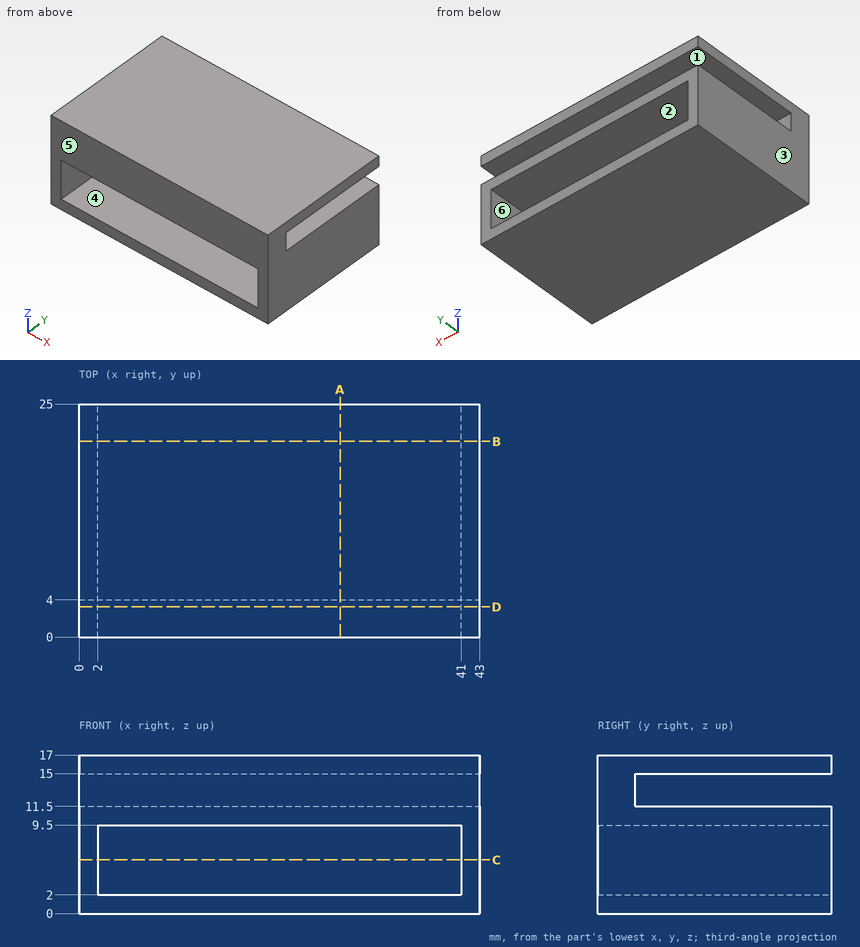
Geometry: see drawing. Coordinates: mm, zero at the bounding-box minimum. A direction names the side the tool comes from. Coordinates: 2 decimals unless noted, no trailing zeros. Loops run counter-clockwise (first coordinate to the right, second up) from the corner with the lowest first, then second, coordinate; pieces in that order, holes last.
(1) Section B-B on y = 21. Return the cut outline in (x, z), then the cut area to 3 significant figures.
(2) Set-up query: the marked faces 5 and 6. Return all of +Z, -Z, +X, -X, +Y, -Y with unobstructed straight access to the full face (end or side cutting, diameter ignored); none if empty.
(3) Pull-direction query (X, two-part tool) for the marked faces 1, 2, 3 and 4; classes: released by +X, released by -X, zero draft, split by the parting line, or undercut.
(4) Section D-D on y = 3.25. Return the cut outline in (x, z), then the cut area to 4 significant figures.
(5) First-contact query: pin 1 Ø2 at (x, z) = (15, 4.5) entering from +Y; pin 2 Ø10 at (x, z) = (19.5, 10) entering from -Y. Flat tips, straight axial feed; report the tip coordinate or a pass-through.
(6) Section C-C on z = 5.75. Return the cut outline in (x, y), then the cut area to 3 significant figures.
(7) Material intervals for probe 1 along Z at (x, y) = (13.5, 5.75); probe 2 along Z at (x, y) = (41.5, 4.5); probe 3 along X at (y, z) = (6.25, 6), sorted ascending.
(8) Section A-A on x = 28. Return the cut outline in (y, z), then the cut area to 3 significant figures.
Data:
1. outline: (0, 0) - (43, 0) - (43, 11.5) - (0, 11.5) - close; (0, 15) - (43, 15) - (43, 17) - (0, 17) - close; hole (2, 2) - (41, 2) - (41, 9.5) - (2, 9.5) - close
1. area: 288 mm2
2. face 5: +Z, -Z, +X, -X, -Y
2. face 6: +Y, -Y
3. face 1: zero draft
3. face 2: undercut
3. face 3: released by -X
3. face 4: undercut
4. outline: (0, 0) - (43, 0) - (43, 17) - (0, 17) - close; hole (2, 2) - (41, 2) - (41, 9.5) - (2, 9.5) - close
4. area: 438.5 mm2
5. pin 1: passes through
5. pin 2: stops at y = 0
6. outline: (0, 0) - (2, 0) - (2, 25) - (0, 25) - close; (41, 0) - (43, 0) - (43, 25) - (41, 25) - close
6. area: 100 mm2
7. probe 1: z = 0 to 2, 9.5 to 11.5, 15 to 17
7. probe 2: z = 0 to 11.5, 15 to 17
7. probe 3: x = 0 to 2, 41 to 43
8. outline: (0, 0) - (25, 0) - (25, 2) - (0, 2) - close; (0, 9.5) - (25, 9.5) - (25, 11.5) - (4, 11.5) - (4, 15) - (25, 15) - (25, 17) - (0, 17) - close
8. area: 164 mm2
